Read the model definition and answer for the solid it produces. Units are mm, in the model's axes. Face numbers are marked on the shaded views. A direction names the side the tool comes from. Give positions to 0.01 mm unless a question says otherwise; leave off trailing zeros. Use a Markdown table: item, result. Add a question column.
Item 1: For the marked faces 1, 2, 3, 4 and 5, determine the directions among +Z, -Z, +X, -X, +Y, -Y from which every point of the face is accessible in a straight line to the end or side of a thin tool.
Item 2: The mould has two halves that part along Y. Classify the marked faces 6, 7 and 8: pulls with the +Y half, pulls with the -Y half, needs draft (parallel to the pull), parting line crosses it, or undercut.
Item 3: Consider probe 1 along X at (y, z) = (-5, 266.5) (1 decimal); probe 2 along Y at (x, z) = (21.5, 146.5); probe 3 along X at (y, z) = (-88.5, 168.5) (1 decimal). Determine where each line is inside the solid, lowest interval first. Write a range as [from, to].
Item 4: A cutting plane is placed at B-B on y = 0. Count the separate pieces of the cut face and the enclosed holes in it, then the cut area to 3 significant figures.
Item 5: Given P1, Ø5, axis at y = -116.5, z = 76, coming from the +X side; P2, Ø1, axis at x = -161.5, y = -22.5, coming from the +Z side; P3, Ø6, axis at x = -28.5, z = 80, coming from the +Y side, each flat-ended and moving along its own axis, determine where each tip first touches the part or whether it passes through.
from build123d import *

# Parameters (mm, degrees)
F0_W     = 365.125
F0_H     = 292.1
F1_DEPTH = 323.85
F2_R     = 25.4
F3_R     = 12.7
F4_T     = -1.5875
F5_R     = 34.925
F6_DEPTH = 365.126
F7_W     = 415.925
F7_H     = 346.075
F8_DEPTH = 88.9
F9_R     = 25.4


with BuildPart() as f1:
    # F0 (on Top) → F1 (new body)
    with BuildSketch(Plane.XY):
        Rectangle(F0_W, F0_H)
    extrude(amount=F1_DEPTH)

    # F2
    f2_edges = [f1.edges().sort_by_distance(p)[0] for p in [
        (-182.5625, -146.05, 161.925),
        (182.5625, -146.05, 161.925),
        (182.5625, 146.05, 161.925),
        (-182.5625, 146.05, 161.925),
    ]]
    fillet(f2_edges, radius=F2_R)

    # F3
    f3_edges = [f1.edges().sort_by_distance(p)[0] for p in [
        (0, -146.05, 0),
    ]]
    fillet(f3_edges, radius=F3_R)

    # F4
    f4_openings = [f1.faces().sort_by_distance(p)[0] for p in [
        (0, 0, 323.85),
    ]]
    offset(amount=F4_T, openings=f4_openings)

    # F5 (on face) → F6 (cut, through all)
    with BuildSketch(Plane.YZ.offset(182.5625)):
        with Locations((0, 66.675)):
            Circle(F5_R)
    extrude(amount=-F6_DEPTH, mode=Mode.SUBTRACT)

    # F7 (on face) → F8 (join)
    with BuildSketch(Plane.XY.offset(323.85)):
        Rectangle(F7_W, F7_H)
        with BuildLine():
            Line((-182.5625, -120.65), (-182.5625, 120.65))
            ThreePointArc((-182.5625, 120.65), (-175.123012, 138.610512), (-157.1625, 146.05))
            Line((-157.1625, 146.05), (157.1625, 146.05))
            ThreePointArc((157.1625, 146.05), (175.123012, 138.610512), (182.5625, 120.65))
            Line((182.5625, 120.65), (182.5625, -120.65))
            ThreePointArc((182.5625, -120.65), (175.123012, -138.610512), (157.1625, -146.05))
            Line((157.1625, -146.05), (-157.1625, -146.05))
            ThreePointArc((-157.1625, -146.05), (-175.123012, -138.610512), (-182.5625, -120.65))
        make_face(mode=Mode.SUBTRACT)
    extrude(amount=-F8_DEPTH)

    # F9
    f9_edges = [f1.edges().sort_by_distance(p)[0] for p in [
        (-207.9625, -173.0375, 279.4),
        (207.9625, -173.0375, 279.4),
        (207.9625, 173.0375, 279.4),
        (-207.9625, 173.0375, 279.4),
    ]]
    fillet(f9_edges, radius=F9_R)


solid = f1.part
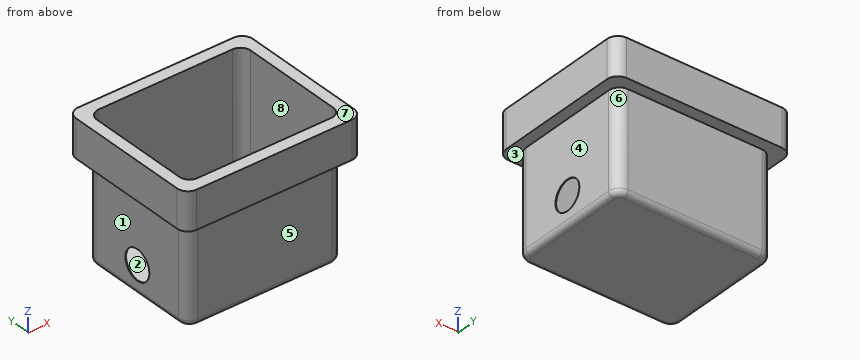
Filled in:
| question | item | result |
|---|---|---|
| 1 | face 1 | -Z, -X, +Y, -Y |
| 1 | face 2 | +Z |
| 1 | face 3 | -Z |
| 1 | face 4 | -Z, +X, +Y, -Y |
| 1 | face 5 | -Z, +X, -X, -Y |
| 2 | face 6 | pulls with the +Y half |
| 2 | face 7 | needs draft |
| 2 | face 8 | undercut |
| 3 | probe 1 | [-208, -181], [181, 208] |
| 3 | probe 2 | [-146.05, -144.46], [144.46, 146.05] |
| 3 | probe 3 | [-182.6, -181], [181, 182.6] |
| 4 | separate pieces | 3 |
| 4 | enclosed holes | 0 |
| 4 | area | 5,880 mm² |
| 5 | P1 | x = 182.56 |
| 5 | P2 | z = 1.59 |
| 5 | P3 | y = 146.05 |
